The model under review builds one solid part; all positions refer to its coordinate system, in mm. Face numbers are marked on the shaded views. A direction names the side the tool comes from. Round coordinates to 2 decimals unless told otherwise and drop trailing zeros. Order: outer loops, then holes, each group sorted by start corner. A loop starts at its lowest first (then second) coordinate and runs counter-clockwise, first axis right, second up. Notation, with made-up numbers: M -23,79.25 L -9,79.25 A10 cw -9,96.25 Z; hole C 6.5,-38 d6. An arc over 180 degrees is marked long. Answer as CSV lines item,"result". Start each with the question number.
Autodesk Inventor part; units mm, degrees
ref_plane "YZ Plane" through (0, 0, 0) normal (1, 0, 0) x (0, 1, 0)
ref_plane "XZ Plane" through (0, 0, 0) normal (0, 1, 0) x (-1, 0, 0)
ref_plane "XY Plane" through (0, 0, 0) normal (0, 0, 1) x (1, 0, 0)
sketch "Sketch2" plane through (0, 0, 0) normal (1, 0, 0) x (0, 1, 0)
  circle A0 centre (100.6118, 121.1829) radius 2.667
  circle A1 centre (62.5118, 121.1829) radius 2.667
  line L0 (100.6118, 121.1829) -> (62.5118, 121.1829) construction
  arc A2 (100.6118, 116.7379) -> (103.3814, 124.6597) centre (100.6118, 121.1829) ccw
  arc A3 (59.0351, 123.9525) -> (62.5118, 116.7379) centre (62.5118, 121.1829) ccw
  line L1 (100.6118, 116.7379) -> (86.6418, 116.7379)
  line L2 (62.5118, 116.7379) -> (67.5918, 116.7379)
  line L3 (67.5918, 116.7379) -> (67.5918, 114.8329)
  line L4 (70.7668, 111.6579) -> (83.4668, 111.6579)
  line L5 (86.6418, 114.8329) -> (86.6418, 116.7379)
  arc A4 (64.8377, 138.2082) -> (96.5877, 138.2082) centre (80.7127, 138.2082) ccw
  line L6 (77.1168, 111.6579) -> (77.1168, 163.1454) construction
  line L7 (99.1277, 138.2082) -> (96.5877, 138.2082)
  line L8 (64.8377, 138.2082) -> (62.2977, 138.2082)
  line L9 (99.1277, 138.2082) -> (99.1277, 128.0482)
  line L10 (99.1277, 128.0482) -> (103.3814, 124.6597)
  line L11 (62.2977, 138.2082) -> (62.2977, 128.0482)
  line L12 (62.2977, 128.0482) -> (59.0351, 123.9525)
  line L13 (99.1277, 128.0482) -> (62.2977, 128.0482) construction
  arc A5 (83.4668, 111.6579) -> (86.6418, 114.8329) centre (83.4668, 114.8329) ccw
  arc A6 (67.5918, 114.8329) -> (70.7668, 111.6579) centre (70.7668, 114.8329) ccw
  point P0 (0, 0)
  point P1 (67.5918, 111.6579)
  point P2 (86.6418, 111.6579)
  dimension "d0" = 5.334
  dimension "d1" = 5.334
  dimension "d2" = 38.1
  dimension "d3" = 8.89
  dimension "d4" = 8.89
  dimension "d7" = 31.75
  dimension "d8" = 9.525
  dimension "d9" = 13.97
  dimension "d10" = 5.08
  dimension "d11" = 2.54
  dimension "d12" = 2.54
  dimension "d13" = 10.16
  dimension "d24" = 3.175
extrude "Extrusion1" add sketch "Sketch2" along normal mid plane 16.002
sketch "Sketch3" plane through (-8.001, 99.1277, 128.0482) normal (0, 1, 0) x (1, 0, 0)
  line L0 (0, 0) -> (0, -10.16)
  line L1 (0, -10.16) -> (16.002, -10.16)
  circle A0 centre (8.001, -7.62) radius 1.27
  point P0 (8.001, 128.0482)
  dimension "d16" = 2.54
  dimension "d17" = 8.001
  dimension "d18" = 2.54
extrude "Extrusion2" cut sketch "Sketch3" against normal up to surface (36.83 mm away)
sketch "Sketch6" plane through (8.001, 70.7668, 111.6579) normal (0, 0, -1) x (-1, 0, 0)
  circle A0 centre (8.001, 6.35) radius 3.175
  line L0 (0, 0) -> (16.002, 12.7) construction
  point P0 (8.001, -70.7668)
  dimension "d25" = 6.35
extrude "Extrusion4" cut sketch "Sketch6" against normal blind 25.4
properties part number "Axle Housing - Front - Custom"
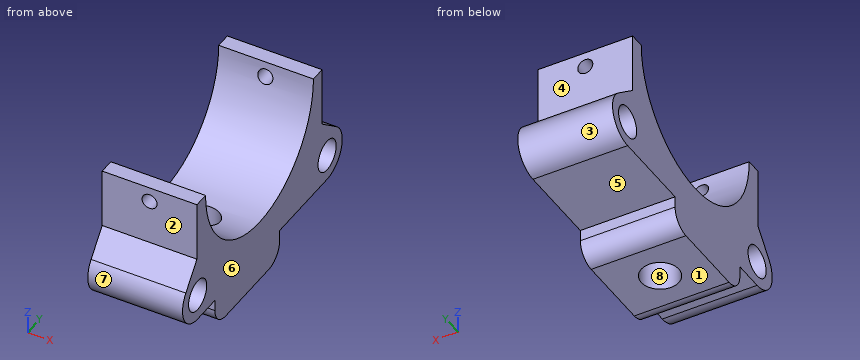
Item 1: The part is to be moulded in two halves that separate along X. For the marked faces 6, 7 and 8, say which applies: +X half, -X half, draft (parallel to the pull), parting line (faces both ways), or undercut.
Item 2: Tool access review of the marked faces 1, 2, 3, 4 and 5: name each direction out of +Z, -Z, +X, -X, +Y, -Y from which nothing blocks a thin tool from reaching the whole face with its end or side.
Item 3: Consider section A-A (y = 101.5). State the section outline as (x, z) points, and give its area (3 significant figures).
Item 4: For pin 1 (3 mm diameter, centred on x = -2.5, z = 131.5, fed in from -Y); pin 2 (1.5 mm diameter, centred on x = 2.5, z = 115.5, fed in from -Y); pin 3 (7.5 mm diameter, centred on x = 0, y = 77.12, fed in from +Z); pin 4 (3 mm diameter, centred on y = 100.61, z = 121.18, fed in from -X), all flat-tipped, find the tip position at first contact; note any pin that passes through.
Item 5: Consider section C-C (z = 126). State the section outline as (x, y) points, and give its area (3 significant figures).
Item 6: Consider section B-B (x = 0). State how many separate pieces and enclosed holes the cut face has, and give its area (3 significant figures).
Item 7: Consider section D-D (z = 135). State the section outline as (x, y) points, and give its area (3 significant figures).
Item 8: Wall thickness on probe 1 along Y at (x, z) = (3.25, 121); probe 2 along Y at (x, z) = (0, 121.25); probe 3 along Z at (x, y) = (-0.75, 98.5): over which ranges is each line inside the solid? List them lowest first. Write a range as [from, to].
Reported:
1,face 6,"+X half"
1,face 7,"draft"
1,face 8,"undercut"
2,face 1,"-Z, +X, -X, +Y, -Y"
2,face 2,"+Z, +X, -X, -Y"
2,face 3,"+X, -X, +Y"
2,face 4,"+Z, +X, -X, +Y"
2,face 5,"-Z, +X, -X, +Y"
3,outline,"M -8,116.83 L 8,116.83 L 8,118.67 L -8,118.67 Z; M -8,123.7 L 8,123.7 L 8,126.16 L -8,126.16 Z"
3,area,"68.8 mm²"
4,pin 1,"stops at y = 62.3"
4,pin 2,"stops at y = 67.59"
4,pin 3,"stops at z = 124.13"
4,pin 4,"passes through"
5,outline,"M -8,60.67 L 8,60.67 L 8,70.57 L -8,70.57 Z; M -8,90.86 L 8,90.86 L 8,101.7 L -8,101.7 Z"
5,area,"332 mm²"
6,separate pieces,"4"
6,enclosed holes,"2"
6,area,"438 mm²"
7,outline,"M -8,62.3 L -1.08,62.3 L -1.08,65.17 L -8,65.17 Z; M -8,96.26 L -1.08,96.26 L -1.08,99.13 L -8,99.13 Z; M 1.08,62.3 L 8,62.3 L 8,65.17 L 1.08,65.17 Z; M 1.08,96.26 L 8,96.26 L 8,99.13 L 1.08,99.13 Z"
7,area,"79.4 mm²"
8,probe 1,"y = [58.07, 59.85], [65.17, 97.95], [103.27, 105.05]"
8,probe 2,"y = [58.07, 59.85], [65.18, 73.94], [80.29, 97.95], [103.28, 105.06]"
8,probe 3,"z = [116.74, 119.55], [122.81, 134.64], [136.69, 138.21]"
